The model under review builds one solid part; all positions refer to its coordinate system, in mm. Give positions to 0.01 mm unless a question says otherwise; leave off trailing zeros. Use CSV: the item, a comma, the result in double quotes. Start each with the question number.
1. Draft analysis for pull direction Z (two halves, no side actions). For faces 1 (the conical face through (-9.88, 2.97, 0.02)), 2 (the conical face through (4.92, -2.97, 8.57)), 3 (the cylindrical face through (5.17, -0.04, -1.15)), state which applies: released by +Z, released by -Z, zero draft, split by the parting line, or undercut.
2. To check wall thickness, follow line 1 (Z direction, x = 0, y = -0.75) (3 decimals); line 2 (X direction, y = -0.75, z = 1); line 3 (X direction, y = -1, z = -0.5). State the ranges of each line that lie inside material, in increasing order. Write a range as [from, to].
3. For pin 1 (1.5 mm diameter, centred on y = -0.5, z = -7, fed in from +X), flat-tipped, find the tip position at first contact; note if it passes through.
Autodesk Inventor part; units mm, degrees
ref_plane "YZ Plane" through (0, 0, 0) normal (1, 0, 0) x (0, 1, 0)
ref_plane "XZ Plane" through (0, 0, 0) normal (0, 1, 0) x (-1, 0, 0)
ref_plane "XY Plane" through (0, 0, 0) normal (0, 0, 1) x (1, 0, 0)
sketch "Sketch3" plane through (0, 0, 0) normal (0, 1, 0) x (-1, 0, 0)
  line L0 (10.9985, 0) -> (5.4993, -9.525)
  line L1 (5.4993, -9.525) -> (-5.4993, -9.525)
  line L2 (-5.4993, -9.525) -> (-10.9985, 0)
  line L3 (-10.9985, 0) -> (-5.4993, 9.525)
  line L4 (-5.4993, 9.525) -> (5.4993, 9.525)
  line L5 (5.4993, 9.525) -> (10.9985, 0)
  point P0 (0, 0)
  point P1 (0, 0)
  point P2 (0, 0)
  dimension "d27" = 19.05
extrude "Extrusion2" add sketch "Sketch3" along normal mid plane 6.35
sketch "Sketch5" plane through (0, 0, 0) normal (0, 0, 1) x (1, 0, 0)
  line L0 (0, -8.89) -> (0, 8.89)
  line L1 (10.9985, 3.175) -> (5.4993, 3.175) construction
  line L2 (5.4993, 3.175) -> (5.4993, -3.175)
  line L3 (10.9985, 3.175) -> (5.4993, 3.175)
  line L4 (10.9985, 3.175) -> (10.9985, -3.175) construction
  line L5 (5.4993, -3.175) -> (10.9985, -3.175)
  line L6 (9.525, 3.175) -> (10.9985, 3.175)
  line L7 (10.9985, 3.175) -> (10.9985, 2.3243)
  line L8 (10.9985, 2.3243) -> (9.525, 3.175)
  line L9 (0, 0) -> (14.3088, 0) construction
  line L10 (9.525, -3.175) -> (10.9985, -3.175)
  line L11 (10.9985, -3.175) -> (10.9985, -2.3243)
  line L12 (10.9985, -2.3243) -> (9.525, -3.175)
  dimension "d15" = 19.05
  dimension "d16" = 30
revolve "Revolution3" cut sketch "Sketch5" angle 360 about axis through (0, -10, 0) along (0, 1, 0)
hole "Hole1" at (0, 3.175, 0) direction (0, -1, 0) diameter 10.5918 end through all
equation "\"diameter\" = 25.4"
equation "\"length\" = 76.2"
properties part number "Door Plate Nut" material "Steel, Carbon"
Determined:
1,face 1,"split by the parting line"
1,face 2,"released by +Z"
1,face 3,"undercut"
2,line 1,"z = [-9.525, -5.296], [5.296, 9.525]"
2,line 2,"x = [-10.42, -5.2], [5.2, 10.42]"
2,line 3,"x = [-10.71, -5.27], [5.27, 10.71]"
3,pin 1,"stops at x = 7.39"
